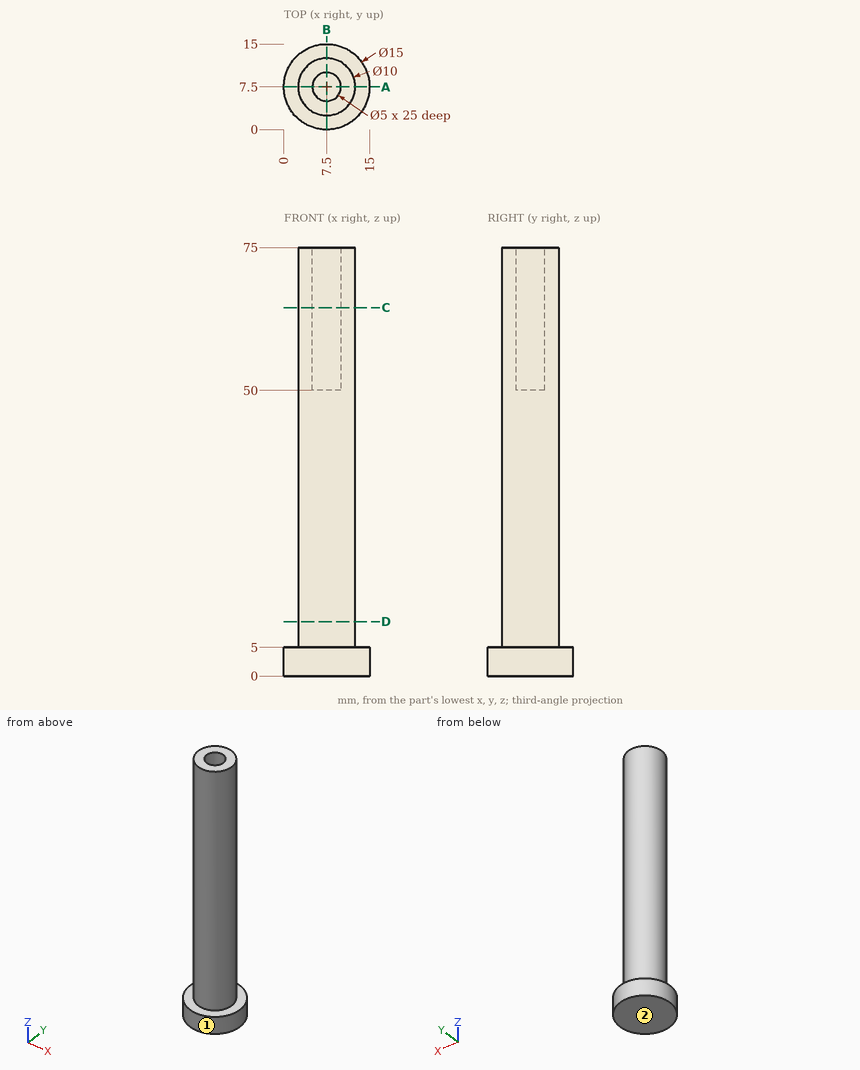
The figure shows three views and two pictorial views of one solid part (mm, origin at its lowest corner). Answer the questions. Give positions to 0.01 mm unless a question says otherwise; leave off trailing zeros. Loops run counter-clockwise (first coordinate to the right, second up) from the corner with the lowest first, then second, coordinate; pieces in that order, holes last. Notation, with made-up numbers: (-34.75, -12) - (5.25, -12) arc R17 cw to (5.25, 17) - close; hole circle Ø1 at (48, 71.25). An arc over 180 degrees is marked (long way). Use one line per item in the form item = value.
1. Find the intervals of material crossed by line 1 along Y through (x, z) = (7.5, 56); line 2 along Y through (x, z) = (7.75, 43.5); line 3 along Z through (x, y) = (1.75, 5.5), in increasing order. Write a range as [from, to].
Calculated:
line_1 = [2.5, 5], [10, 12.5]
line_2 = [2.51, 12.49]
line_3 = [0, 5]
2. Given pin 1 Ø8 at (x, z) = (8, 22) entering from +Y; pin 2 Ø2 at (x, z) = (9.5, 56) entering from -Y; pin 3 Ø1 at (x, z) = (9.5, 41.5) entering from -Y, each flat-ended and moving along its own axis, determine where each tip first touches the part or whether it passes through.
Calculated:
pin_1 = 12.5
pin_2 = 2.6
pin_3 = 2.73
3. Section A-A on y = 7.5 is taken. Give the vertices of the cut face in (x, z), then the cut area to 3 significant figures.
Calculated:
outline = (0, 0) - (15, 0) - (15, 5) - (12.5, 5) - (12.5, 75) - (10, 75) - (10, 50) - (5, 50) - (5, 75) - (2.5, 75) - (2.5, 5) - (0, 5) - close
area = 650 mm^2
4. Section C-C on z = 64.5 is taken. Give the vertices of the cut face in (x, y), then the cut area to 3 significant figures.
Calculated:
outline = circle Ø10 at (7.5, 7.5); hole circle Ø5 at (7.5, 7.5)
area = 58.9 mm^2
5. Section D-D on z = 9.5 is taken. Give the vertices of the cut face in (x, y), then the cut area to 3 significant figures.
Calculated:
outline = circle Ø10 at (7.5, 7.5)
area = 78.5 mm^2
6. The mould has two halves that part along X. Classify the marked faces 1 and 2: pulls with the +X half, pulls with the -X half, needs draft (parallel to the pull), parting line crosses it, or undercut.
Calculated:
face_1 = parting line crosses it
face_2 = needs draft
